For this review, take the finished solid that the model builds, in its own axes (mm). Face numbers are marked on the shaded views. Round coordinates to 2 decimals unless told otherwise and drop trailing zeros. Order: outer loops, then holes, each group sorted by start corner. A loop starts at its lowest first (then second) coordinate and runs counter-clockwise, first axis right, second up. Notation, with made-up numbers: M 51,33 L 70,33 A35 ccw 70,71 Z; hole C -2,58 d10. An arc over 180 degrees is marked long. Answer in a Markdown table with one row per item. Add a question column.
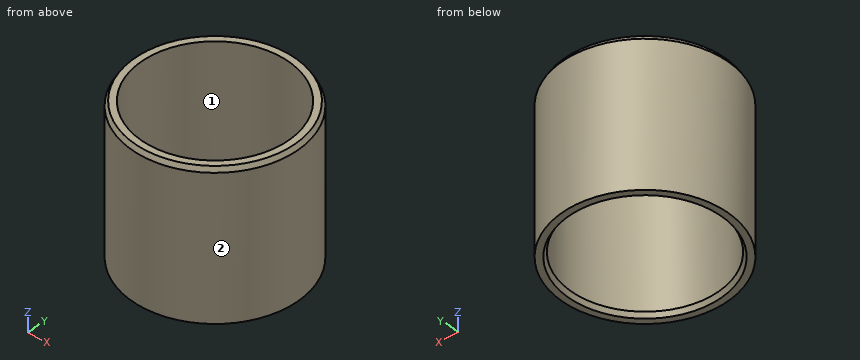
Autodesk Inventor part; units mm, degrees
ref_plane "YZ Plane" through (0, 0, 0) normal (1, 0, 0) x (0, 1, 0)
ref_plane "XZ Plane" through (0, 0, 0) normal (0, 1, 0) x (-1, 0, 0)
ref_plane "XY Plane" through (0, 0, 0) normal (0, 0, 1) x (1, 0, 0)
sketch "Sketch1" plane through (0, 0, 0) normal (0, 0, 1) x (1, 0, 0)
  circle A0 centre (0, 0) radius 14.2875
  dimension "d0" = 28.575
extrude "Body" add sketch "Sketch1" along normal blind 25.4
hole "Hole" at (0, 0, 25.4) direction (0, 0, -1) diameter 25.4 end through all
chamfer "Chamfer - Outside" distance 0.7874 angle 30 1 edges at (-14.2875, 0, 25.4) measured on face at (14.2412, -1.1497, 16.9333)
chamfer "Chamfer - Inside" distance 0.7874 angle 30 1 edges at (0, 12.7, 0) measured on face at (1.0219, -12.6588, 16.9333)
properties part number "JSI-1618-16" material "iglide J"
1. The part is to be moulded in two halves that separate along X. For the marked faces 1 and 2, say which applies: pulls with the +X half, pulls with the -X half, needs draft (parallel to the pull), parting line crosses it, or undercut.
2. Consider section C-C on z = 11.5. Write out the cut boundary in (x, y) (1 decimal).
3. Consider section A-A on x = 0. Write out the cut boundary in (y, z), plus the area to 3 significant figures.
4. Clearance check with flat-ended pins moving along their axes: pin 1 Ø2 at (x, z) = (-5.5, 14) entering from +Y; pin 2 Ø1.5 at (x, z) = (9.5, 3) entering from +Y; pin 3 Ø5 at (x, z) = (7.5, 15.5) entering from +Y. State where each tip first meets the part, or that it passes through.
5. To check wall thickness, follow probe 1 along Y at (x, z) = (0, 11); probe 2 along Y at (x, z) = (-8.5, 8). State the ranges of each line that lie inside material, in increasing order. Write a range as [from, to].
Solved:
| question | item | result |
|---|---|---|
| 1 | face 1 | undercut |
| 1 | face 2 | parting line crosses it |
| 2 | outline | C 0,0 d28.6; hole C 0,0 d25.4 |
| 3 | outline | M -14.29,0 L -13.15,0 L -12.7,0.79 L -12.7,25.4 L -13.83,25.4 L -14.29,24.61 Z; M 12.7,0.79 L 13.15,0 L 14.29,0 L 14.29,24.61 L 13.83,25.4 L 12.7,25.4 Z |
| 3 | area | 79.9 mm^2 |
| 4 | pin 1 | stops at y = 13.56 |
| 4 | pin 2 | stops at y = 11.29 |
| 4 | pin 3 | stops at y = 13.38 |
| 5 | probe 1 | y = [-14.29, -12.7], [12.7, 14.29] |
| 5 | probe 2 | y = [-11.48, -9.44], [9.44, 11.48] |
